For this review, use the dimensioned drawing (mm, ordinates from the lowest corner) and the shaded views. A direction names the side the tool comes from. Coordinates: 2 decimals unless noted, no trailing zeros. Write each loop counter-clockwise with the first axis right and the second up, starting at its lowest first coordinate (ties: lowest second). Pieces come first, ordered by that corner, then holes. Notation, with made-up numbers: (29.25, 0.5) - (72.25, 0.5) arc R35 cw to (72.25, 32.5) - close; hole circle Ø7 at (52.5, 48). An arc over 180 degrees is marked (long way). Answer as a JSON object with one key per item and string values.
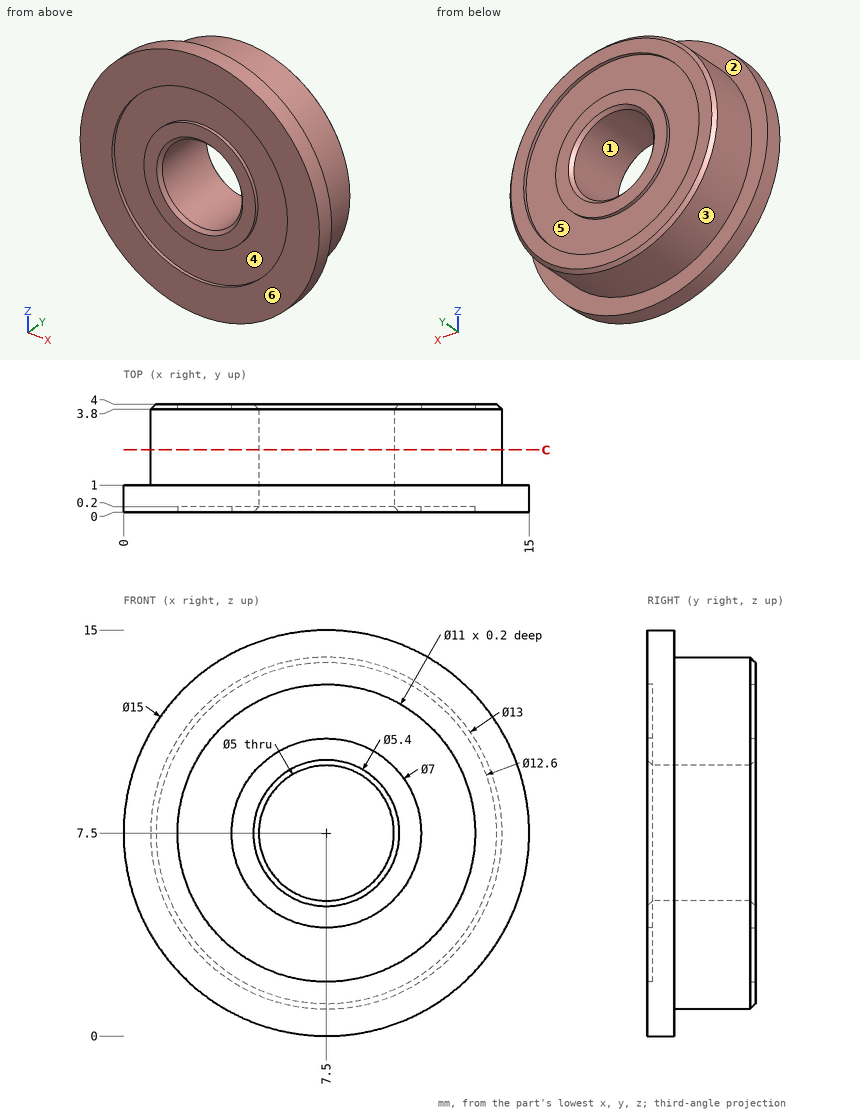
(1) To check wall thickness, follow line 1 (Z direction, x = 7.5, y = 1.05); line 2 (X direction, y = 3.9, z = 7.5); line 3 (X direction, y = 0.1, z = 7.5). State the ranges of each line that lie inside material, in increasing order. Write a range as from..to.
Solved:
{"line 1": "z = 1..5, 10..14", "line 2": "x = 1.1..2, 4..4.9, 10.1..11, 13..13.9", "line 3": "x = 0..2, 4..4.9, 10.1..11, 13..15"}
(2) The part is to be moulded in two halves that separate along Z. For the marked faces 1, 2 and 3, say which applies: pulls with the +Z half, pulls with the -Z half, needs draft (parallel to the pull), parting line crosses it, or undercut.
Solved:
{"face 1": "undercut", "face 2": "needs draft", "face 3": "parting line crosses it"}
(3) Tool access review of the marked faces 4, 5 and 6: name each direction out of +Z, -Z, +X, -X, +Y, -Y from which nothing blocks a thin tool from reaching the whole face with its end or side.
Solved:
{"face 4": "-Y", "face 5": "+Y", "face 6": "+Z, -Z, +X, -X, -Y"}
(4) For pin 1 (1 mm diameter, centred on y = 2, z = 13.5, fed in from +X); pin 2 (6.5 mm diameter, centred on x = 7.5, z = 7.5, fed in from -Y); pin 3 (1.5 mm diameter, centred on y = 3, z = 13, fed in from -X); pin 4 (1 mm diameter, centred on x = 12, y = 2, fed in from -Z), all flat-tipped, find the tip position at first contact; note any pin that passes through.
Solved:
{"pin 1": "stops at x = 10.96", "pin 2": "stops at y = 0", "pin 3": "stops at x = 3.06", "pin 4": "stops at z = 2.38"}
(5) Take a section at C-C, the plane y = 2.3. Write out the cut boundary in (x, z).
Solved:
{"outline": "circle Ø13 at (7.5, 7.5); hole circle Ø5 at (7.5, 7.5)"}
